```python
from build123d import *

# Parameters (mm, degrees)
SKETCH_1_R                       = 3.6
SKETCH_1_R_2                     = 1.25
SM_BASE_FLANGE_1_DEPTH           = 2
SM_EDGE_FLANGE_1_STRIP_W         = 9.4732
SM_EDGE_FLANGE_1_STRIP_H         = 2
SM_EDGE_FLANGE_1_STRIP_CUT_DEPTH = 25
SM_EDGE_FLANGE_1_DEPTH           = 25
SM_EDGE_FLANGE_1_PROFILE_W       = 25
SM_EDGE_FLANGE_1_PROFILE_H       = 24.2634
SM_EDGE_FLANGE_1_PROFILE_R       = 2.1
SM_EDGE_FLANGE_1_PROFILE_R_2     = 5
SM_EDGE_FLANGE_1_FLAT_DEPTH      = 2


# Sheet-metal steps are written as plain solids
with BuildPart() as part:
    # Sketch 1 → 基体-法兰1 (new body)
    with BuildSketch(Plane.XY):
        with BuildLine():
            Line((12.5, 0), (-12.5, 0))
            Line((-12.5, 0), (-12.5, 18))
            ThreePointArc((-12.5, 18), (0, 30.5), (12.5, 18))
            Line((12.5, 18), (12.5, 0))
        make_face()
        with Locations((0, 18)):
            Circle(SKETCH_1_R, mode=Mode.SUBTRACT)
        with Locations((-8.5, 18)):
            Circle(SKETCH_1_R_2, mode=Mode.SUBTRACT)
        with Locations(Location((8.5, 18, 0), (0, 0, 180))):
            Circle(SKETCH_1_R_2, mode=Mode.SUBTRACT)
    extrude(amount=-SM_BASE_FLANGE_1_DEPTH)

    # 边线-法兰1 strip (across the edge) → 边线-法兰1 strip cut (cut)
    with BuildSketch(Plane.YZ.offset(-12.5)):
        with Locations((-2, -1)):
            Rectangle(SM_EDGE_FLANGE_1_STRIP_W, SM_EDGE_FLANGE_1_STRIP_H)
    extrude(amount=SM_EDGE_FLANGE_1_STRIP_CUT_DEPTH, mode=Mode.SUBTRACT)

    # 边线-法兰1 bend section (across the edge) → 边线-法兰1 (add)
    with BuildSketch(Plane.YZ.offset(-12.5)):
        with BuildLine():
            Line((0, 0.7366), (2, 0.7366))
            ThreePointArc((2, 0.7366), (2.215745145, 0.215745145), (2.7366, 0))
            Line((2.7366, 0), (2.7366, -2))
            ThreePointArc((2.7366, -2), (0.801531583, -1.198468417), (0, 0.7366))
        make_face()
    extrude(amount=SM_EDGE_FLANGE_1_DEPTH)

    # 边线-法兰1 profile (on flange) → 边线-法兰1 flat (add)
    with BuildSketch(Plane.XZ):
        with Locations((0, 12.8683)):
            Rectangle(SM_EDGE_FLANGE_1_PROFILE_W, SM_EDGE_FLANGE_1_PROFILE_H)
        with Locations((-7.425, 5.075)):
            Circle(SM_EDGE_FLANGE_1_PROFILE_R, mode=Mode.SUBTRACT)
        with Locations((7.425, 5.075)):
            Circle(SM_EDGE_FLANGE_1_PROFILE_R, mode=Mode.SUBTRACT)
        with Locations((-7.425, 19.925)):
            Circle(SM_EDGE_FLANGE_1_PROFILE_R, mode=Mode.SUBTRACT)
        with Locations((0, 12.5)):
            Circle(SM_EDGE_FLANGE_1_PROFILE_R_2, mode=Mode.SUBTRACT)
        with Locations((7.425, 19.925)):
            Circle(SM_EDGE_FLANGE_1_PROFILE_R, mode=Mode.SUBTRACT)
    extrude(amount=-SM_EDGE_FLANGE_1_FLAT_DEPTH)


solid = part.part
```
Source: CAD feature listing. Evaluate the final solid. Frame: model axes, mm. A direction names the side the tool comes from. Round coordinates to 2 decimals unless told otherwise and drop trailing zeros. Loops run counter-clockwise (first coordinate to the right, second up) from the corner with the lowest first, then second, coordinate; pieces in that order, holes last. Notation, with made-up numbers: M 60,51.5 L 66,51.5 A31 cw 66,76.5 Z; hole C 59,87 d1. An arc over 180 degrees is marked long. Use a Markdown table: item, result. Add a question column.
1. Section query B-B on x = -8.5. Return the cut outline in (y, z), then the cut area to 3 significant figures.
2. Section query C-C on z = 21.25. Return the cut outline in (x, y), then the cut area to 3 significant figures.
3. Section query A-A on z = 12.5. Return the cut outline in (x, y).
4. Contact query for flat-ended pins moving along their axis: P1, Ø4, axis at x = -7.425, z = 19.925, coming from the +Y side; P2, Ø10, axis at y = 4.5, z = 9, coming from the +X side; P3, Ø3, axis at x = -8.5, y = 18, coming from the +Z side; P4, Ø5, axis at x = -7.425, z = 5.075, coming from the +Y side. Output: stop coordinate, or through.
5. Line query: line 1 (Z direction, x = -3.75, y = 3); line 2 (Y direction, x = -8.75, z = 21.75); line 3 (Z direction, x = 0, y = 1.2). Output: solid intervals per line, ascending.
6. Reachability of faces 1 (the flat face through (-12.5, 1.6, 5.4)), 2 (the flat face through (0, 2, 18)) from +Z, -Z, +X, -X, +Y, -Y: full face, straight path, thin tool, end or side. Return the list, or none.
7. Mould query, pull axis Y, two halves, no side actions, for faces 3 (the cylindrical face through (-5.485, 0.986, 19.121)), 4 (the cylindrical face through (-0.78, 14.486, -0.986)), 5 (the cylindrical face through (9.421, 17.155, -0.986)), 6 (the cylindrical face through (-0.175, 0.823, -1.22)). Classes: pulls with the +Y half, pulls with the -Y half, needs draft (parallel to the pull), parting line crosses it, or undercut.
8. Section query D-D on y = 15. Return the cut outline in (x, z), then the cut area to 3 significant figures.
Reported:
| question | item | result |
|---|---|---|
| 1 | outline | M 0,0.74 A2.74 ccw 2.74,-2 L 16.75,-2 L 16.75,0 L 2.74,0 A0.74 cw 2,0.74 L 2,3.27 L 0,3.27 Z; M 0,6.88 L 2,6.88 L 2,18.12 L 0,18.12 Z; M 0,21.73 L 2,21.73 L 2,25 L 0,25 Z; M 19.25,-2 L 27.17,-2 L 27.17,0 L 19.25,0 Z |
| 1 | area | 83.4 mm² |
| 2 | outline | M -12.5,0 L -9.05,0 L -9.05,2 L -12.5,2 Z; M -5.8,0 L 5.8,0 L 5.8,2 L -5.8,2 Z; M 9.05,0 L 12.5,0 L 12.5,2 L 9.05,2 Z |
| 2 | area | 37.0 mm² |
| 3 | outline | M -12.5,0 L -5,0 L -5,2 L -12.5,2 Z; M 5,0 L 12.5,0 L 12.5,2 L 5,2 Z |
| 4 | P1 | passes through |
| 4 | P2 | stops at x = 12.5 |
| 4 | P3 | stops at z = 0 |
| 4 | P4 | stops at y = 2 |
| 5 | line 1 | z = -2 to 0 |
| 5 | line 2 | y = 0 to 2 |
| 5 | line 3 | z = -1.53 to 7.5, 17.5 to 25 |
| 6 | face 1 | +Z, -Z, -X, +Y, -Y |
| 6 | face 2 | +Z, +X, -X, +Y |
| 7 | face 3 | needs draft |
| 7 | face 4 | undercut |
| 7 | face 5 | undercut |
| 7 | face 6 | pulls with the -Y half |
| 8 | outline | M -12.5,-2 L -1.99,-2 L -1.99,0 L -12.5,0 Z; M 1.99,-2 L 12.5,-2 L 12.5,0 L 1.99,0 Z |
| 8 | area | 42.0 mm² |
